Verification items for the finished model (mm, model axes). Face numbers are marked on the shaded views. Round coordinates to 2 decimals unless told otherwise and drop trailing zeros. Write each loop counter-clockwise with the first axis right and the second up, starting at its lowest first coordinate (ties: lowest second). Pieces come first, ordered by that corner, then holes. Notation, with made-up numbers: M 42,55 L 71,55 A14 cw 71,61 Z; hole C 89,70.5 d10. An arc over 180 degrees is marked long. One line per question, with ' | ' between items. Start each with the question number.
Q1. Cross-section at A-A (x = 0). Record the boundary of the cut face in (y, z).
Q2. Cross-section at B-B (z = 0). Record the boundary of the cut face in (x, y), then the cut area to 3 significant figures.
Q3. Cross-section at C-C (y = -27.5). Record the boundary of the cut face in (x, z), then the cut area to 3 significant figures.
Q4. Release check for a two-part mould opening along Z. For the marked faces 1 and 2 record: released by +Z, released by -Z, zero draft, split by the parting line, or undercut.
Q5. Gauge pin test, flat ends, axial feed: pin 1 (1 mm diameter, centred on y = -21, z = 15.5, fed in from +X); pin 2 (10 mm diameter, centred on y = -12.5, z = 20.5, fed in from -X); pin 3 (12 mm diameter, centred on x = 12, z = -19.5, fed in from -Y). Record the tip position at first contact, or that the pin passes through.
Q6. Thickness scan on line 1 along Z through (x, y) = (0, -2.1); line 2 along Y through (x, z) = (1, -2.5); line 3 along Z through (x, y) = (0, -31.5). Record the ranges inside material, lowest first. Write a range as from..to.
Q7. Cross-section at D-D (x = -6). Record the boundary of the cut face in (y, z), then the cut area to 3 significant figures.
from build123d import *

# Parameters (mm, degrees)
F1_R     = 19.05
F2_DEPTH = 25
F3_R     = 2.1
F4_DEPTH = 3
F5_R     = 2
F6_DEPTH = 25


with BuildPart() as f2:
    # F1 (on offset) → F2 (new body)
    with BuildSketch(Plane.XZ):
        Circle(F1_R)
    extrude(amount=F2_DEPTH)

    # F3 (on offset) → F4 (join)
    with BuildSketch(Plane.XZ):
        with BuildLine():
            ThreePointArc((4.828854, 25), (0, 29.828854), (-4.828854, 25))
            Line((-4.828854, 25), (-4.828854, 18.427823))
            ThreePointArc((-4.828854, 18.427823), (0, 19.05), (4.828854, 18.427823))
            Line((4.828854, 18.427823), (4.828854, 25))
        make_face()
        with Locations((0, 25)):
            Circle(F3_R, mode=Mode.SUBTRACT)
        with BuildLine():
            ThreePointArc((-4.828854, -25), (0, -29.828854), (4.828854, -25))
            Line((4.828854, -25), (4.828854, -18.427823))
            ThreePointArc((4.828854, -18.427823), (0, -19.05), (-4.828854, -18.427823))
            Line((-4.828854, -18.427823), (-4.828854, -25))
        make_face()
        with Locations((0, -25)):
            Circle(F3_R, mode=Mode.SUBTRACT)
    extrude(amount=F4_DEPTH)

    # F5 (on face) → F6 (join)
    with BuildSketch(Plane.XZ.offset(25)):
        Circle(F5_R)
    extrude(amount=F6_DEPTH)


solid = f2.part
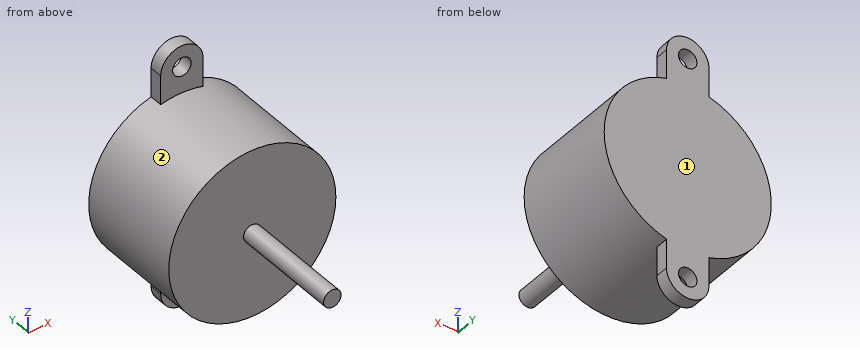
Determined:
1) outline: M -50,-2 L -25,-2 L -25,-19.05 L -3,-19.05 L -3,-22.9 L 0,-22.9 L 0,22.9 L -3,22.9 L -3,19.05 L -25,19.05 L -25,2 L -50,2 Z; M -3,-29.83 L 0,-29.83 L 0,-27.1 L -3,-27.1 Z; M -3,27.1 L 0,27.1 L 0,29.83 L -3,29.83 Z
2) outline: M -19.05,-25 L -2,-25 L -2,-50 L 2,-50 L 2,-25 L 19.05,-25 L 19.05,0 L -19.05,0 Z | area: 1,050 mm²
3) outline: C 0,0 d4 | area: 12.6 mm²
4) face 1: zero draft | face 2: split by the parting line
5) pin 1: stops at x = 11.74 | pin 2: stops at x = -11.07 | pin 3: stops at y = -25
6) line 1: z = -29.83..-27.1, -22.9..22.9, 27.1..29.83 | line 2: y = -25..0 | line 3: z = -2..2
7) outline: M -25,-18.08 L 0,-18.08 L 0,18.08 L -25,18.08 Z | area: 904 mm²
